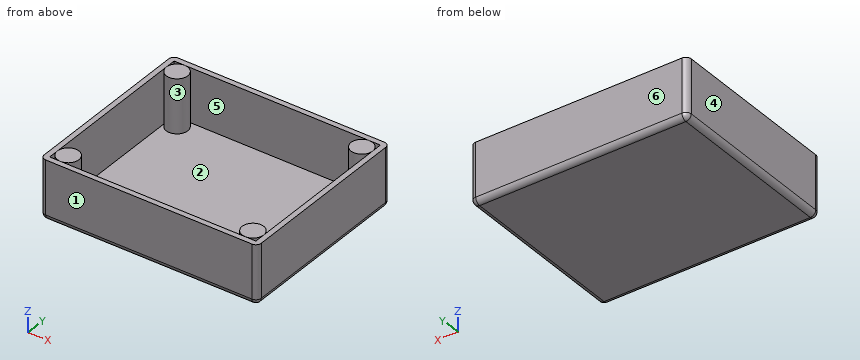
from build123d import *

# Parameters (mm, degrees)
SKETCH_W     = 38.36735
SKETCH_H     = 31.836736
PAD_DEPTH    = 10
THICKNESS_T  = 1
SKETCH001_R  = 2
PAD001_DEPTH = 10


with BuildPart() as part:
    # Sketch → Pad (new body)
    with BuildSketch(Plane.XY):
        with Locations((-0.408164, 1.632655)):
            Rectangle(SKETCH_W, SKETCH_H)
    extrude(amount=PAD_DEPTH)

    # Thickness
    thickness_openings = [part.faces().sort_by_distance(p)[0] for p in [
        (-0.408164, 1.632655, 10),
    ]]
    offset(amount=THICKNESS_T, openings=thickness_openings)

    # Sketch001 (on Face5 of Thickness) → Pad001 (join)
    with BuildSketch(Plane.XY):
        with Locations((-17.591839, 15.551023)):
            Circle(SKETCH001_R)
        with Locations((16.775511, 15.551023)):
            Circle(SKETCH001_R)
        with Locations((16.775511, -12.285713)):
            Circle(SKETCH001_R)
        with Locations((-17.591839, -12.285713)):
            Circle(SKETCH001_R)
    extrude(amount=PAD001_DEPTH)


solid = part.part
The model under review builds one solid part; all positions refer to its coordinate system, in mm. Face numbers are marked on the shaded views. A direction names the side the tool comes from. Round coordinates to 2 decimals unless told otherwise and drop trailing zeros. Loops run counter-clockwise (first coordinate to the right, second up) from the corner with the lowest first, then second, coordinate; pieces in that order, holes last. Notation, with made-up numbers: M 26.5,41 L 44.5,41 A32 cw 44.5,72 Z; hole C 6,22 d3. An arc over 180 degrees is marked long. Answer as CSV lines item,"result". Start each with the question number.
Item 1: Wall thickness on line 1 (X direction, y = -4, z = 9); line 2 (Y direction, x = -13, z = 8.75); line 3 (Y direction, x = 15.5, z = 3.5): over which ranges is each line inside the solid? List them lowest first. Write a range as [from, to].
Item 2: Consider section B-B (y = 2.5). Write out the cut boundary in (x, z), then the cut area to 3 significant figures.
Item 3: Consider section D-D (x = -16.5). Write out the cut boundary in (y, z), then the cut area to 3 significant figures.
Item 4: Mouldability with a two-part tool opening along X and no side actions: class the marked faces 3, 4, 5 and 6 as released by +X, released by -X, zero draft, split by the parting line, or undercut.
Item 5: For the marked faces 1 and 2, list the 3-axis set-ups (+Z, -Z, +X, -X, +Y, -Y) from which the entire face can be reached by the end or side of a thin tool; tool diameter is ignored.
Item 6: Insertion check: P1, Ø1.5, axis at x = 8.5, y = 4, coming from the +Z side. The pin has a flat end and moves straight along its axis. Give the tip position at first contact, or say it passes through.
Item 7: Consider section C-C (x = 14). Write out the cut boundary in (y, z).
Answer:
1,line 1,"x = [-20.59, -19.59], [18.78, 19.78]"
1,line 2,"y = [-15.29, -14.29], [17.55, 18.55]"
1,line 3,"y = [-15.29, -14.29], [-13.83, -10.75], [14.01, 17.09], [17.55, 18.55]"
2,outline,"M -20.59,0 A1 ccw -19.59,-1 L 18.78,-1 A1 ccw 19.78,0 L 19.78,10 L 18.78,10 L 18.78,0 L -19.59,0 L -19.59,10 L -20.59,10 Z"
2,area,"59.9 mm^2"
3,outline,"M -15.29,0 A1 ccw -14.29,-1 L 17.55,-1 A1 ccw 18.55,0 L 18.55,10 L 17.55,10 L 17.55,0 L 17.23,0 L 17.23,10 L 13.88,10 L 13.88,0 L -10.61,0 L -10.61,10 L -13.96,10 L -13.96,0 L -14.29,0 L -14.29,10 L -15.29,10 Z"
3,area,"120 mm^2"
4,face 3,"undercut"
4,face 4,"released by -X"
4,face 5,"undercut"
4,face 6,"zero draft"
5,face 1,"+Z, -Z, +X, -X, -Y"
5,face 2,"+Z"
6,P1,"stops at z = 0"
7,outline,"M -15.29,0 A1 ccw -14.29,-1 L 17.55,-1 A1 ccw 18.55,0 L 18.55,10 L 17.55,10 L 17.55,0 L -14.29,0 L -14.29,10 L -15.29,10 Z"
